Can you work these out from the model? Positions are in its coordinate system, mm. A direction names the side the tool comes from. Give positions to 0.01 mm unless a question says otherwise; leave off trailing zeros. Order: outer loops, then holes, each group sorted by start corner. A loop starts at its lowest first (then second) coordinate and runs counter-clockwise, first axis right, second up. Notation, with made-up numbers: M 71.25,70 L 126.25,70 A25 cw 126.25,93 Z; hole C 51.5,66 d11. An arc over 180 degrees is marked long. Use a Markdown table: item, result. Add a question column.
from build123d import *

# Parameters (mm, degrees)
F0_W     = 90
F0_H     = 35
F1_DEPTH = 5
F3_R     = 15
F2_W     = 2
F2_H     = 33
F4_DEPTH = 90
F5_W     = 30
F5_H     = 35
F6_DEPTH = 1.5


with BuildPart() as f1:
    # F0 (on Front) → F1 (new body)
    with BuildSketch(Plane.XZ):
        with Locations((-2.3338645697, 1.2048181861)):
            Rectangle(F0_W, F0_H)
    extrude(amount=F1_DEPTH)

    # F3
    f3_edges = [f1.edges().sort_by_distance(p)[0] for p in [
        (42.666135, -2.5, -16.295182),
        (-47.333865, -2.5, -16.295182),
    ]]
    fillet(f3_edges, radius=F3_R)

    # F2 (on face) → F4 (cut)
    with BuildSketch(Plane(origin=(-47.3338645697, 0, 0), x_dir=(0, -1, 0), z_dir=(-1, 0, 0))):
        with Locations((2.5, 0.2048181861)):
            Rectangle(F2_W, F2_H)
    extrude(amount=-F4_DEPTH, mode=Mode.SUBTRACT)

    # F5 (on face) → F6 (cut)
    with BuildSketch(Plane.XZ.offset(5)):
        with Locations((2.6661354303, 1.2048181861)):
            Rectangle(F5_W, F5_H)
    extrude(amount=-F6_DEPTH, mode=Mode.SUBTRACT)


solid = f1.part
1. On a 3-axis mill with a long thin cutter (end or side, diameter ignored), from which of +Z, -Z, +X, -X, +Y, -Y can I reach the whole of each face in a straight line? I mean faces 1 (the face through (-12.334, -4, 1)), 2 (the face through (-43.06, -0.76, -11.78)), 3 (the face through (-3, -2, 16.705)). Say none if no direction works.
2. Will these pins go through, and if not, where does the flat tip stop? pin 1 (1 mm diameter, centred on x = 2.5, z = 18, fed in from -Y); pin 2 (1.5 mm diameter, centred on x = 6.5, z = -4, fed in from -Y).
3. I need wall thicknesses on L1, parallel to Y at x = 26.5, z = -13; L2, parallel to X at y = -4.4, z = 5; L3, parallel to Z at x = 21.5, y = -1.6. Which ranges of each line are inside material? Lowest first, please. Write a range as [from, to].
4. If we section it at C-C, the plane z = -7: List the corners of the cut face in (x, y) for me.
5. If we section it at A-A, the plane z = 0: List the corners of the cut face in (x, y) for me, then the cut area to 3 significant figures.
6. If we section it at D-D, the plane x = -19: List the corners of the cut face in (y, z) for me.
7. If we section it at B-B, the plane x = 6: List the corners of the cut face in (y, z) for me.
Geometry results:
| question | item | result |
|---|---|---|
| 1 | face 1 | +Z, -Z, -Y |
| 1 | face 2 | -Z, -X, +Y, -Y |
| 1 | face 3 | -Z, +X, -X |
| 2 | pin 1 | stops at y = -3.5 |
| 2 | pin 2 | stops at y = -1.5 |
| 3 | L1 | y = [-5, -3.5], [-1.5, 0] |
| 3 | L2 | x = [-47.33, -12.33], [17.67, 42.67] |
| 3 | L3 | z = [16.7, 18.7] |
| 4 | outline | M -46.21,-5 L -12.33,-5 L -12.33,-3.5 L -46.21,-3.5 Z; M -46.21,-1.5 L 41.54,-1.5 L 41.54,0 L -46.21,0 Z; M 17.67,-5 L 41.54,-5 L 41.54,-3.5 L 17.67,-3.5 Z |
| 5 | outline | M -47.33,-5 L -12.33,-5 L -12.33,-3.5 L -47.33,-3.5 Z; M -47.33,-1.5 L 42.67,-1.5 L 42.67,0 L -47.33,0 Z; M 17.67,-5 L 42.67,-5 L 42.67,-3.5 L 17.67,-3.5 Z |
| 5 | area | 225 mm^2 |
| 6 | outline | M -5,-16.3 L -3.5,-16.3 L -3.5,16.7 L -1.5,16.7 L -1.5,-16.3 L 0,-16.3 L 0,18.7 L -5,18.7 Z |
| 7 | outline | M -3.5,16.7 L -1.5,16.7 L -1.5,-16.3 L 0,-16.3 L 0,18.7 L -3.5,18.7 Z |
